Design review of the part built by this model. Coordinates are the model's own, in mm. A direction names the side the tool comes from. Give positions to 0.01 mm unless a question says otherwise; leave off trailing zeros. Loops run counter-clockwise (first coordinate to the right, second up) from the corner with the lowest first, then second, coordinate; pieces in that order, holes last. Notation, with made-up numbers: M -23.75,-4 L -12.75,-4 A19 cw -12.75,8 Z; hole C -31.5,27.25 d2. An arc over 180 degrees is marked long. Answer as CSV lines item,"result".
```python
from build123d import *
from build123d import SkipClean  # not in build123d's __all__

# Parameters (mm, degrees)
F2_R     = 2.5
F2_W     = 17.5
F2_H     = 8.8
F3_DEPTH = 15
F4_R     = 2.5
F4_W     = 17.5
F4_H     = 8.8
F5_DEPTH = 1.8


with BuildPart() as f3:
    # F2 (on Top) → F3 (new body)
    with BuildSketch(Plane.XY):
        with BuildLine():
            ThreePointArc((-13.7742425586, -3.6791308501), (-12.2542853153, -2.1117815941), (-11.7, 0))
            ThreePointArc((-11.7, 0), (-12.2542853153, 2.1117815941), (-13.7742425586, 3.6791308501))
            ThreePointArc((-13.7742425586, 3.6791308501), (-20.3, 0), (-13.7742425586, -3.6791308501))
        make_face()
        with Locations((-16, 0)):
            Circle(F2_R, mode=Mode.SUBTRACT)
        with BuildLine():
            ThreePointArc((-13.7742425586, 3.6791308501), (-12.2542853153, 2.1117815941), (-11.7, 0))
            ThreePointArc((-11.7, 0), (-12.2542853153, -2.1117815941), (-13.7742425586, -3.6791308501))
            Line((-13.7742425586, -3.6791308501), (-12.4064937305, -6.2))
            Line((-12.4064937305, -6.2), (0, -6.2))
            Line((0, -6.2), (12.4064937305, -6.2))
            Line((12.4064937305, -6.2), (13.913982062, -3.7601235568))
            ThreePointArc((13.913982062, -3.7601235568), (11.7, 0), (13.913982062, 3.7601235568))
            Line((13.913982062, 3.7601235568), (12.4064937305, 6.2))
            Line((12.4064937305, 6.2), (0, 6.2))
            Line((0, 6.2), (-12.4064937305, 6.2))
            Line((-12.4064937305, 6.2), (-13.7742425586, 3.6791308501))
        make_face()
        Rectangle(F2_W, F2_H, mode=Mode.SUBTRACT)
        with BuildLine():
            ThreePointArc((20.3, 0), (18.1817565019, 3.705393173), (13.913982062, 3.7601235568))
            ThreePointArc((13.913982062, 3.7601235568), (11.7, 0), (13.913982062, -3.7601235568))
            ThreePointArc((13.913982062, -3.7601235568), (18.1817565019, -3.705393173), (20.3, 0))
        make_face()
        with Locations((16, 0)):
            Circle(F2_R, mode=Mode.SUBTRACT)
    extrude(amount=F3_DEPTH)

    # F4 (on face) → F5 (join)
    with BuildSketch(Plane(origin=(0, 0, 0), x_dir=(1, 0, 0), z_dir=(0, 0, -1))):
        with BuildLine():
            Line((-12.4064937305, 6.2), (-13.7742425586, 3.6791308501))
            ThreePointArc((-13.7742425586, 3.6791308501), (-20.3, 0), (-13.7742425586, -3.6791308501))
            Line((-13.7742425586, -3.6791308501), (-12.4064937305, -6.2))
            Line((-12.4064937305, -6.2), (12.4064937305, -6.2))
            Line((12.4064937305, -6.2), (13.913982062, -3.7601235568))
            ThreePointArc((13.913982062, -3.7601235568), (20.3, 0), (13.913982062, 3.7601235568))
            Line((13.913982062, 3.7601235568), (12.4064937305, 6.2))
            Line((12.4064937305, 6.2), (-12.4064937305, 6.2))
        make_face()
        with Locations((-16, 0)):
            Circle(F4_R, mode=Mode.SUBTRACT)
        Rectangle(F4_W, F4_H, mode=Mode.SUBTRACT)
        with Locations((16, 0)):
            Circle(F4_R, mode=Mode.SUBTRACT)
        Rectangle(F4_W, F4_H)
    with SkipClean():  # cleaning this boolean's faces spoils the solid; the shape is the same uncleaned
        extrude(amount=F5_DEPTH)


solid = f3.part
```
1. For faces 1 (the flat face through (0, 4.4, 7)), 2 (the flat face through (0, 0, -1.8)), list the 3-axis set-ups (+Z, -Z, +X, -X, +Y, -Y) from which the entire face can be reached by the end or side of a thin tool; tool diameter is ignored.
Answer block:
face 1,"+Z"
face 2,"-Z, +X, -X, +Y, -Y"
2. We need section B-B, the plane z = 1. Write out the cut boundary in (x, y), plus the area to 3 significant figures.
Answer block:
outline,"M -13.77,-3.68 L -12.41,-6.2 L 12.41,-6.2 L 13.91,-3.76 A4.3 ccw long 13.91,3.76 L 12.41,6.2 L -12.41,6.2 L -13.77,3.68 A4.3 ccw long Z; hole C -16,0 d5; hole M -8.75,-4.4 L 8.75,-4.4 L 8.75,4.4 L -8.75,4.4 Z; hole C 16,0 d5"
area,"236 mm²"
3. We need section A-A, the plane x = -16. Write out the cut boundary in (y, z).
Answer block:
outline,"M -4.3,-1.8 L -2.5,-1.8 L -2.5,15 L -4.3,15 Z; M 2.5,-1.8 L 4.3,-1.8 L 4.3,15 L 2.5,15 Z"
4. We need section D-D, the plane x = 4. Write out the cut boundary in (y, z), plus the area to 3 significant figures.
Answer block:
outline,"M -6.2,-1.8 L 6.2,-1.8 L 6.2,15 L 4.4,15 L 4.4,0 L -4.4,0 L -4.4,15 L -6.2,15 Z"
area,"76.3 mm²"
5. We need section C-C, the plane y = -1.25. Write out the cut boundary in (x, z).
Answer block:
outline,"M -20.11,-1.8 L -18.17,-1.8 L -18.17,15 L -20.11,15 Z; M -13.83,-1.8 L 13.83,-1.8 L 13.83,15 L 8.75,15 L 8.75,0 L -8.75,0 L -8.75,15 L -13.83,15 Z; M 18.17,-1.8 L 20.11,-1.8 L 20.11,15 L 18.17,15 Z"
6. To check wall thickness, follow L1, parallel to X at y = 0, z = -1.35; L2, parallel to Y at x = -5.5, z = 6.5; L3, parallel to Y at x = 16, z = 9. State the ranges of each line that lie inside material, in increasing order. Write a range as [from, to].
Answer block:
L1,"[-20.3, -18.5], [-13.5, 13.5], [18.5, 20.3]"
L2,"[-6.2, -4.4], [4.4, 6.2]"
L3,"[-4.3, -2.5], [2.5, 4.3]"
7. The part is to be moulded in two halves that separate along Y. For faces 3 (the flat face through (0, 0, 0)), 4 (the flat face through (0, 6, 15)), say which applies: pulls with the +Y half, pulls with the -Y half, needs draft (parallel to the pull), parting line crosses it, or undercut.
Answer block:
face 3,"undercut"
face 4,"needs draft"
8. For P1, Ø4.5, axis at x = 16, y = 0, coming from the +Z side; P2, Ø1, axis at x = 1, y = 1, coming from the +Z side; P3, Ø2, axis at y = -4.5, z = 1, coming from the +X side; P4, Ø1.5, axis at y = -3, z = 6, coming from the +X side, all flat-tipped, find the tip position at first contact; note any pin that passes through.
Answer block:
P1,"through"
P2,"z = 0"
P3,"x = 18.5"
P4,"x = 19.66"
